Source: CAD feature listing. Evaluate the final solid. Frame: model axes, mm. A direction names the side the tool comes from. Give positions to 0.01 mm unless a question says otherwise; leave off trailing zeros. Loops run counter-clockwise (first coordinate to the right, second up) from the corner with the lowest first, then second, coordinate; pieces in that order, holes last.
from build123d import *

# Parameters (mm, degrees)
F0_W      = 63.5
F0_H      = 38.1
F1_DEPTH  = 6.35
F2_W      = 50.8
F2_H      = 19.05
F3_DEPTH  = 19.05
F4_W      = 38.1
F4_H      = 11.938
F5_DEPTH  = 19.05
F6_R      = 5.08
F7_W      = 31.75
F7_H      = 19.05
F8_DEPTH  = 19.05
F9_R      = 12.446
F10_DEPTH = 25.401


with BuildPart() as f1:
    # F0 (on Top) → F1 (new body)
    with BuildSketch(Plane.XY):
        Rectangle(F0_W, F0_H)
    extrude(amount=F1_DEPTH)

    # F2 (on face) → F3 (join)
    with BuildSketch(Plane.XY.offset(6.35)):
        with Locations((-0.093382, 9.525)):
            Rectangle(F2_W, F2_H)
    extrude(amount=F3_DEPTH)

    # F4 (on face) → F5 (cut)
    with BuildSketch(Plane.XY.offset(25.4)):
        with Locations((-0.18145, 13.081)):
            Rectangle(F4_W, F4_H)
    extrude(amount=-F5_DEPTH, mode=Mode.SUBTRACT)

    # F6
    f6_edges = [f1.edges().sort_by_distance(p)[0] for p in [
        (-31.75, -19.05, 3.175),
        (31.75, -19.05, 3.175),
    ]]
    fillet(f6_edges, radius=F6_R)

    # F7 (on face) → F8 (join)
    with BuildSketch(Plane.XY.offset(6.35)):
        with Locations((-1.774265, -9.525)):
            Rectangle(F7_W, F7_H)
    extrude(amount=F8_DEPTH)

    # F9 (on face) → F10 (cut, through all)
    with BuildSketch(Plane.XY.offset(25.4)):
        with Locations((-1.774265, -19.05)):
            Circle(F9_R)
    extrude(amount=-F10_DEPTH, mode=Mode.SUBTRACT)


solid = f1.part
1) Pull-direction query (X, two-part tool) for faces 6 (the flat face through (14.101, -10, 16)), 7 (the flat face through (-19.231, 13, 16)), 8 (the cylindrical face through (-30.301, -17.522, 3.219)); classes: released by +X, released by -X, zero draft, split by the parting line, or undercut.
Checks:
face 6: released by +X
face 7: undercut
face 8: released by -X
2) Cut plane C-C (x = -22.5). Return loops of the section in (y, z), and give its area (3 significant figures).
Checks:
outline: (-19.05, 0) - (19.05, 0) - (19.05, 25.4) - (0, 25.4) - (0, 6.35) - (-19.05, 6.35) - close
area: 605 mm2
3) Ray query, probe 1 along X at (y, z) = (11, 12.5); probe 2 along Z at (x, y) = (-22.5, -13.5); probe 3 along Y at (x, z) = (-15.5, 12.5). Return the intervals inside material, ascending.
Checks:
probe 1: x = -25.49 to -19.23, 18.87 to 25.31
probe 2: z = 0 to 6.35
probe 3: y = -19.05 to 7.11
4) Reachability of faces 1 (the flat face through (18.869, 13, 16)), 2 (the flat face through (31.75, 2, 3)), 3 (the flat face through (-25.493, 9, 16)), 4 (the flat face through (-22, 0, 16)), 5 (the flat face through (25.307, 9, 16)) from +Z, -Z, +X, -X, +Y, -Y: full face, straight path, thin tool, end or side. Return the list, or none.
Checks:
face 1: +Z, +Y
face 2: +Z, -Z, +X, +Y, -Y
face 3: +Z, -X, +Y, -Y
face 4: +Z, -X, -Y
face 5: +Z, +X, +Y, -Y
5) Cut plane D-D (z = 4). Return loops of the section in (x, y).
Checks:
outline: (-31.75, -13.97) arc R5.08 ccw to (-26.67, -19.05) - (-14.22, -19.05) arc R12.45 cw to (10.67, -19.05) - (26.67, -19.05) arc R5.08 ccw to (31.75, -13.97) - (31.75, 19.05) - (-31.75, 19.05) - close
6) Cut plane B-B (y = 1). Return loops of the section in (x, z).
Checks:
outline: (-31.75, 0) - (31.75, 0) - (31.75, 6.35) - (25.31, 6.35) - (25.31, 25.4) - (-25.49, 25.4) - (-25.49, 6.35) - (-31.75, 6.35) - close
7) Contact query for flat-ended pins moving along their axis: P1, Ø15, axis at y = -12, z = 19, coming from the +X side; P2, Ø6, axis at x = -7.5, y = 13, coming from the +Z side; P3, Ø5.5, axis at x = 17.5, z = 12, coming from the -Y side. Output: stop coordinate, or through.
Checks:
P1: stops at x = 14.1
P2: stops at z = 6.35
P3: stops at y = 0
